Could you check a few things on this drawing? It's one solid part, dimensions in mm from its lowest x, y, z. Coordinates: 2 decimals unless noted, no trailing zeros. Order: outer loops, then holes, each group sorted by start corner. A loop starts at its lowest first (then second) coordinate and runs counter-clockwise, first axis right, second up. Notation, with made-up numbers: (9, 65.25) -> (34, 65.25) arc R26 ccw to (34, 79.25) -> close; hole circle Ø4 at (40.5, 88.5). An arc over 180 degrees is marked (long way). Use a Markdown table: item, result. Add a question column.
1. Suppose I cut it at A-A, the plane z = 40. List the corners of the cut face in (x, y) for me.
2. If I drill on line 1 along Z through (x, y) = (158, 1.35); line 2 along X through (y, z) = (1.3, 21); line 3 along X through (y, z) = (0.4, 21.5), over which ranges is the centre line in solid material (lowest first)? Write a range as from..to.
3. Suppose I cut it at C-C, the plane y = 1.1. List the corners of the cut face in (x, z) for me.
4. Suppose I cut it at D-D, the plane z = 20. List the corners of the cut face in (x, y) for me, then the cut area to 3 significant figures.
5. Suppose I cut it at B-B, the plane x = 158. List the corners of the cut face in (y, z) for me.
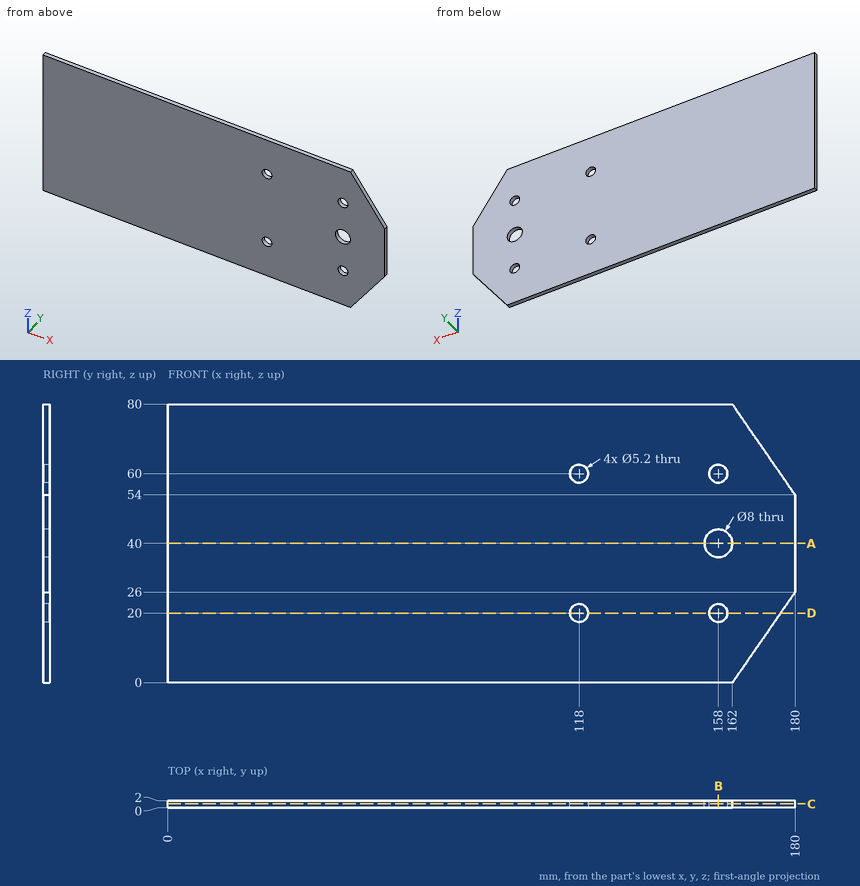
Worked out:
| question | item | result |
|---|---|---|
| 1 | outline | (0, 0) -> (154, 0) -> (154, 2) -> (0, 2) -> close; (162, 0) -> (180, 0) -> (180, 2) -> (162, 2) -> close |
| 2 | line 1 | z = 0..17.4, 22.6..36, 44..57.4, 62.6..80 |
| 2 | line 2 | x = 0..115.6, 120.4..155.6, 160.4..176.54 |
| 2 | line 3 | x = 0..115.88, 120.12..155.88, 160.12..176.88 |
| 3 | outline | (0, 0) -> (162, 0) -> (180, 26) -> (180, 54) -> (162, 80) -> (0, 80) -> close; hole circle Ø5.2 at (118, 20); hole circle Ø5.2 at (118, 60); hole circle Ø8 at (158, 40); hole circle Ø5.2 at (158, 20); hole circle Ø5.2 at (158, 60) |
| 4 | outline | (0, 0) -> (115.4, 0) -> (115.4, 2) -> (0, 2) -> close; (120.6, 0) -> (155.4, 0) -> (155.4, 2) -> (120.6, 2) -> close; (160.6, 0) -> (175.85, 0) -> (175.85, 2) -> (160.6, 2) -> close |
| 4 | area | 331 mm² |
| 5 | outline | (0, 0) -> (2, 0) -> (2, 17.4) -> (0, 17.4) -> close; (0, 22.6) -> (2, 22.6) -> (2, 36) -> (0, 36) -> close; (0, 44) -> (2, 44) -> (2, 57.4) -> (0, 57.4) -> close; (0, 62.6) -> (2, 62.6) -> (2, 80) -> (0, 80) -> close |
